```python
from build123d import *

# Parameters (mm, degrees)
SKETCH_W      = 107
SKETCH_H      = 72
PAD_DEPTH     = 2
SKETCH001_W   = 1
SKETCH001_H   = 64
PAD001_DEPTH  = 3
SKETCH002_W   = 1
SKETCH002_H   = 64
PAD002_DEPTH  = 2
SKETCH003_W   = 1
SKETCH003_H   = 64
PAD003_DEPTH  = 2
SKETCH004_W   = 1
SKETCH004_H   = 64
PAD004_DEPTH  = 3
SKETCH005_W   = 99
SKETCH005_H   = 1
PAD005_DEPTH  = 3
SKETCH006_W   = 99
SKETCH006_H   = 1
PAD006_DEPTH  = 2
SKETCH007_W   = 99
SKETCH007_H   = 1
PAD007_DEPTH  = 2
SKETCH008_W   = 99
SKETCH008_H   = 1
PAD008_DEPTH  = 3
SKETCH009_R   = 23.5
SKETCH009_R_2 = 2
SKETCH009_R_3 = 1
SKETCH009_W   = 27.757637
SKETCH009_H   = 31.122207
POCKET_DEPTH  = 2.001


with BuildPart() as part:
    # Sketch → Pad (new body)
    with BuildSketch(Plane.XY):
        with Locations((53.5, 36)):
            Rectangle(SKETCH_W, SKETCH_H)
    extrude(amount=-PAD_DEPTH)

    # Sketch001 → Pad001 (join)
    with BuildSketch(Plane.XY):
        with Locations((0.5, 36)):
            Rectangle(SKETCH001_W, SKETCH001_H)
    extrude(amount=PAD001_DEPTH)

    # Sketch002 → Pad002 (join)
    with BuildSketch(Plane.XY):
        with Locations((3, 36)):
            Rectangle(SKETCH002_W, SKETCH002_H)
    extrude(amount=PAD002_DEPTH)

    # Sketch003 → Pad003 (join)
    with BuildSketch(Plane.XY):
        with Locations((104, 36)):
            Rectangle(SKETCH003_W, SKETCH003_H)
    extrude(amount=PAD003_DEPTH)

    # Sketch004 → Pad004 (join)
    with BuildSketch(Plane.XY):
        with Locations((106.5, 36)):
            Rectangle(SKETCH004_W, SKETCH004_H)
    extrude(amount=PAD004_DEPTH)

    # Sketch005 → Pad005 (join)
    with BuildSketch(Plane.XY):
        with Locations((53.5, 71.5)):
            Rectangle(SKETCH005_W, SKETCH005_H)
    extrude(amount=PAD005_DEPTH)

    # Sketch006 → Pad006 (join)
    with BuildSketch(Plane.XY):
        with Locations((53.5, 69)):
            Rectangle(SKETCH006_W, SKETCH006_H)
    extrude(amount=PAD006_DEPTH)

    # Sketch007 → Pad007 (join)
    with BuildSketch(Plane.XY):
        with Locations((53.5, 3)):
            Rectangle(SKETCH007_W, SKETCH007_H)
    extrude(amount=PAD007_DEPTH)

    # Sketch008 → Pad008 (join)
    with BuildSketch(Plane.XY):
        with Locations((53.5, 0.5)):
            Rectangle(SKETCH008_W, SKETCH008_H)
    extrude(amount=PAD008_DEPTH)

    # Sketch009 → Pocket (cut, through all)
    with BuildSketch(Plane.XY):
        with Locations((31.773752, 37.38124)):
            Circle(SKETCH009_R)
        with Locations((12.328316, 56.826676)):
            Circle(SKETCH009_R_2)
        with Locations((51.219189, 56.826676)):
            Circle(SKETCH009_R_2)
        with Locations((51.219189, 17.935803)):
            Circle(SKETCH009_R_2)
        with Locations((12.328316, 17.935803)):
            Circle(SKETCH009_R_2)
        with Locations((63.572306, 58.290639)):
            Circle(SKETCH009_R_3)
        with Locations((98.572306, 58.290639)):
            Circle(SKETCH009_R_3)
        with Locations((63.572306, 18.290639)):
            Circle(SKETCH009_R_3)
        with Locations((98.572306, 18.290639)):
            Circle(SKETCH009_R_3)
        with BuildLine():
            ThreePointArc((78.061318, 11.354568), (76.210807, 9.504057), (78.061318, 7.653547))
            Line((78.061318, 7.653547), (93.874763, 7.653547))
            ThreePointArc((93.874763, 7.653547), (95.725274, 9.504057), (93.874763, 11.354568))
            Line((78.061318, 11.354568), (93.874763, 11.354568))
        make_face()
        with Locations((81.173542, 38.523415)):
            Rectangle(SKETCH009_W, SKETCH009_H)
    extrude(amount=-POCKET_DEPTH, mode=Mode.SUBTRACT)


solid = part.part
```
Model file for the job. Use its own axes, mm. A direction names the side the tool comes from. Coordinates: 2 decimals unless noted, no trailing zeros. Write each loop counter-clockwise with the first axis right and the second up, starting at its lowest first coordinate (ties: lowest second). Pieces come first, ordered by that corner, then holes. Notation, with made-up numbers: (73.25, -30) - (123.25, -30) arc R16 ccw to (123.25, -23) - close; hole circle Ø3 at (49, -3.5). An arc over 180 degrees is marked (long way). One line per item, written item: value. Start each with the question number.
1. Slice it at C-C (y = 44). Write the cut outline in (x, z).
2. Flat gauge pins, fed straight in: pin 1 (2 mm diameter, centred on y = 42, z = 0.5, fed in from -X); pin 2 (4 mm diameter, centred on x = 74, y = 11.5, fed in from +Z); pin 3 (0.5 mm diameter, centred on x = 3, y = 31, fed in from +Z); pin 4 (0.8 mm diameter, centred on y = 0.5, z = 1, fed in from +X). Where does each tip first touch, or does it go through?
3. Tool access for faces 1 (the flat face through (106, 36, 1)), 2 (the cylindrical face through (76.21, 9.54, -0.99)), 3 (the flat face through (53, 3.5, 1)), 4 (the flat face through (107, 35, 1)): list every direction of +Z, -Z, +X, -X, +Y, -Y with a clear straight run to the whole face (end or side of a thin tool).
4. Mould opens along Y. For faces 5 (the flat face through (104.5, 36, 1)), 6 (the flat face through (81, 54.085, -1)), 7 (the flat face through (53, 72, 1)) say: released by +Y, released by -Y, zero draft, split by the parting line, or undercut.
5. Slice it at D-D (y = 6.5). Write the cut outline in (x, z).
6. Slice it at A-A (z = 1). Count the separate pieces of the cut face and the enclosed holes in it, plus the area to 3 significant figures.
7. Slice it at B-B (x = 73.5). Write the cut outline in (y, z), plus the area to 3 significant figures.
8. Probe line 1 (X direction, y = 20.5, z = 1.3); line 2 (Y direction, x = 52, z = 1.2); line 3 (Y direction, x = 63.5, z = -0.9). List the from-to ranges inside material, lowest first. Write a range as from..to.
Answers below:
1. outline: (0, -2) - (9.23, -2) - (9.23, 0) - (3.5, 0) - (3.5, 2) - (2.5, 2) - (2.5, 0) - (1, 0) - (1, 3) - (0, 3) - close; (54.32, -2) - (67.29, -2) - (67.29, 0) - (54.32, 0) - close; (95.05, -2) - (107, -2) - (107, 3) - (106, 3) - (106, 0) - (104.5, 0) - (104.5, 2) - (103.5, 2) - (103.5, 0) - (95.05, 0) - close
2. pin 1: stops at x = 0
2. pin 2: stops at z = 0
2. pin 3: stops at z = 2
2. pin 4: stops at x = 103
3. face 1: +Z, +Y, -Y
3. face 2: +Z, -Z
3. face 3: +Z, +X, -X
3. face 4: +Z, -Z, +X, +Y, -Y
4. face 5: zero draft
4. face 6: undercut
4. face 7: released by +Y
5. outline: (0, -2) - (107, -2) - (107, 3) - (106, 3) - (106, 0) - (104.5, 0) - (104.5, 2) - (103.5, 2) - (103.5, 0) - (3.5, 0) - (3.5, 2) - (2.5, 2) - (2.5, 0) - (1, 0) - (1, 3) - (0, 3) - close
6. separate pieces: 8
6. enclosed holes: 0
6. area: 652 mm^2
7. outline: (0, -2) - (22.96, -2) - (22.96, 0) - (3.5, 0) - (3.5, 2) - (2.5, 2) - (2.5, 0) - (1, 0) - (1, 3) - (0, 3) - close; (54.08, -2) - (72, -2) - (72, 3) - (71, 3) - (71, 0) - (69.5, 0) - (69.5, 2) - (68.5, 2) - (68.5, 0) - (54.08, 0) - close
7. area: 91.8 mm^2
8. line 1: x = 0..1, 2.5..3.5, 103.5..104.5, 106..107
8. line 2: y = 0..1, 2.5..3.5, 68.5..69.5, 71..72
8. line 3: y = 0..17.29, 19.29..57.29, 59.29..72
